```python
from build123d import *

# Parameters (mm, degrees)
SKETCH1_W           = 20
SKETCH1_H           = 20
BOSS_EXTRUDE1_DEPTH = 500
CUT_EXTRUDE2_DEPTH  = 500
CIRPATTERN1_COUNT   = 4
CUT_EXTRUDE3_REACH  = 502
SKETCH3_R           = 2.1
CUT_EXTRUDE4_DEPTH  = 500
CIRPATTERN2_COUNT   = 4
FILLET1_R           = 3


with BuildPart() as part:
    # Sketch1 → Boss-Extrude1 (new body)
    with BuildSketch(Plane.XY):
        Rectangle(SKETCH1_W, SKETCH1_H)
    extrude(amount=-BOSS_EXTRUDE1_DEPTH)

    # Sketch2 → Cut-Extrude2 (cut)
    with BuildSketch(Plane.XY):
        Polygon((-5.499339828, -6.56), (-2.84, -3.900660172), (2.84, -3.900660172), (5.499339828, -6.56), (5.499339828, -8.2), (2.84, -8.2), (4.64, -10), (-4.64, -10), (-2.84, -8.2), (-5.499339828, -8.2), align=None)
    cut_extrude2 = extrude(amount=-CUT_EXTRUDE2_DEPTH, mode=Mode.SUBTRACT)

    # CirPattern1: Cut-Extrude2 ×4 about axis
    cirpattern1_axis = Axis((0, 0, 0), (0, 0, 1))
    for i in range(1, CIRPATTERN1_COUNT):
        add(cut_extrude2.rotate(cirpattern1_axis, i * 360 / CIRPATTERN1_COUNT), mode=Mode.SUBTRACT)

    # Sketch3 → Cut-Extrude3 (cut, up to next)
    with BuildSketch(Plane.XY, mode=Mode.PRIVATE) as cut_extrude3_sk1:
        Circle(SKETCH3_R)
    cut_extrude3_tool1 = extrude(cut_extrude3_sk1.sketch, amount=-CUT_EXTRUDE3_REACH, mode=Mode.PRIVATE) & part.part
    add(cut_extrude3_tool1.solids().sort_by_distance((0, 0, 0))[0], mode=Mode.SUBTRACT)

    # Sketch4 → Cut-Extrude4 (cut)
    with BuildSketch(Plane.XY):
        Polygon((-8.2, 8.2), (-8.2, 6.569339828), (-6.569339828, 8.2), align=None)
    cut_extrude4 = extrude(amount=-CUT_EXTRUDE4_DEPTH, mode=Mode.SUBTRACT)

    # CirPattern2: Cut-Extrude4 ×4 about axis
    cirpattern2_axis = Axis((0, 0, 0), (0, 0, 1))
    for i in range(1, CIRPATTERN2_COUNT):
        add(cut_extrude4.rotate(cirpattern2_axis, i * 360 / CIRPATTERN2_COUNT), mode=Mode.SUBTRACT)

    # Fillet1
    fillet1_edges = [part.edges().sort_by_distance(p)[0] for p in [
        (10, -10, -250),
        (-10, -10, -250),
        (-10, 10, -250),
        (10, 10, -250),
    ]]
    fillet(fillet1_edges, radius=FILLET1_R)


solid = part.part
```
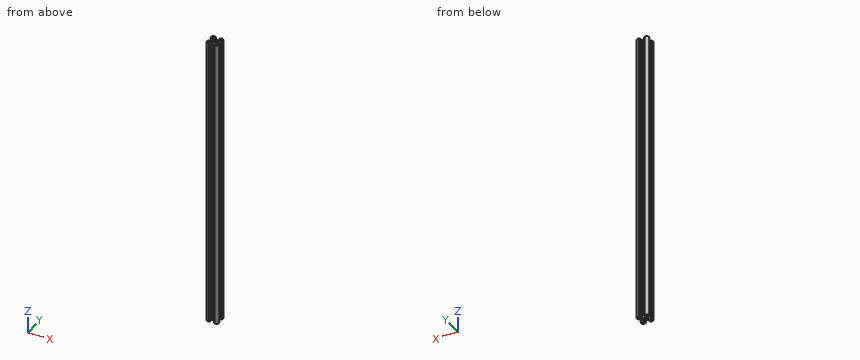
The listing builds one solid part. Answer for the finished solid, in the listing's coordinates (mm). Coordinates: 2 decimals unless noted, no trailing zeros. Write item = value, one per line.
1) Section A-A (z = -72) is taken. Count the separate pieces of the cut face and the enclosed holes in it, plus the area to 3 significant figures.
Responses:
separate_pieces = 1
enclosed_holes = 5
area = 158 mm^2
2) Each of these flat-tipped pins is pushed along its axis until it touches: P1, Ø0.8, axis at y = -4, z = -314, coming from the -X side; P2, Ø6, axis at y = 0.5, z = -342.5, coming from the +X side; P3, Ø2, axis at y = -2.5, z = -329, coming from the -X side. Where does it stop, or does it pass through?
Responses:
P1 = -9.76
P2 = 8.86
P3 = -8.86
3) Find the intervals of material crossed by line 1 along Y through (x, z) = (0, -111.5); line 2 along Y through (x, z) = (8, -117); line 3 along Y through (x, z) = (-3.5, -109.5), in increasing order.
Responses:
line_1 = -3.9 to -2.1, 2.1 to 3.9
line_2 = -9.83 to -8.2, -6.77 to -5.5, 5.5 to 6.77, 8.2 to 9.83
line_3 = -8.86 to -8.2, -4.56 to 4.56, 8.2 to 8.86
